from build123d import *

# Parameters (mm, degrees)
SKETCH1_R           = 4
BOSS_EXTRUDE1_DEPTH = 14
SKETCH2_W           = 12
SKETCH2_H           = 6
CUT_EXTRUDE1_DEPTH  = 17


with BuildPart() as part:
    # Sketch1 → Boss-Extrude1 (new body)
    with BuildSketch(Plane(origin=(0, 0, 0), x_dir=(1, 0, 0), z_dir=(0, 1, 0))):
        with BuildLine():
            Line((-76.999999986, 5.832514168), (-76.999999986, 3.540882964))
            add(Edge.make_bspline(
                [(-6.942295947, 3.975490785), (-13.088937843, 4.53703129), (-37.064176348, 1.721893834), (-62.004711992, -6.566542107), (-76.999999986, 3.540882964)],
                knots=[0.045717223, 0.045717223, 0.045717223, 0.045717223, 0.30042167, 1, 1, 1, 1], degree=3))
            ThreePointArc((-6.942295947, 3.975490785), (4.012235893, -6.921124413), (0, 8))
            add(Edge.make_bspline(
                [(0, 8), (-24.867463869, 10.892678598), (-52.765963903, -4.510038737), (-76.999999986, 5.832514168)],
                knots=[0, 0, 0, 0, 1, 1, 1, 1], degree=3))
        make_face()
        with Locations(Location((0, 0.5, 0), (0, 0, 270))):
            Circle(SKETCH1_R, mode=Mode.SUBTRACT)
    extrude(amount=BOSS_EXTRUDE1_DEPTH)

    # Sketch2 → Cut-Extrude1 (cut, symmetric)
    with BuildSketch(Plane.XY):
        with Locations((2, 7)):
            Rectangle(SKETCH2_W, SKETCH2_H)
    extrude(amount=CUT_EXTRUDE1_DEPTH, both=True, mode=Mode.SUBTRACT)


solid = part.part
CAD build for the part. Positions are in the model's coordinates, mm. A direction names the side the tool comes from. Give positions to 0.01 mm unless a question says otherwise; leave off trailing zeros. Write each question's results on one line, items separated by ' | '.
1. Probe L1, parallel to Z at x = -8.5, y = 4; L2, parallel to Z at x = -32.5, y = 4. List the from-to ranges inside material, lowest first. Write a range as from..to.
Calculated:
L1: z = -8.34..-4.09 | L2: z = -5.22..-1.4
2. 3-axis set-ups, long thin cutter, end or side, ignore diameter. For faces 4 (the face through (5, 10, 0)), 5 (the face through (-25, 0, -3)): which of +Z, -Z, +X, -X, +Y, -Y reach the whole face in a straight line?
Calculated:
face 4: +Z, -Z, +X | face 5: +Z, -Z, +X, -X, -Y
3. Pin check, flat tips, straight feed: pin 1 (2 mm diameter, centred on x = -45, y = 6.5, fed in from -Z); pin 2 (1.5 mm diameter, centred on y = 11.5, z = -2.5, fed in from -X); pin 3 (3 mm diameter, centred on y = 6, z = 0.5, fed in from +X). Stop position of each tip, or through.
Calculated:
pin 1: stops at z = -3.3 | pin 2: stops at x = -76.56 | pin 3: stops at x = -4
4. Saw through at A-A on x = -1.5. Count the separate pieces of the cut face and the enclosed holes in it, and give its area (3 significant figures).
Calculated:
separate pieces: 4 | enclosed holes: 0 | area: 68.8 mm2
5. Pull direction Y, two halves, no side cores. Call faces 1 (the face through (-77, 7, -5)), 2 (the face through (-4, 7, -1)), 3 (the face through (-25, 14, -3)): released by +Y, released by -Y, zero draft, split by the parting line, or undercut.
Calculated:
face 1: zero draft | face 2: undercut | face 3: released by +Y
